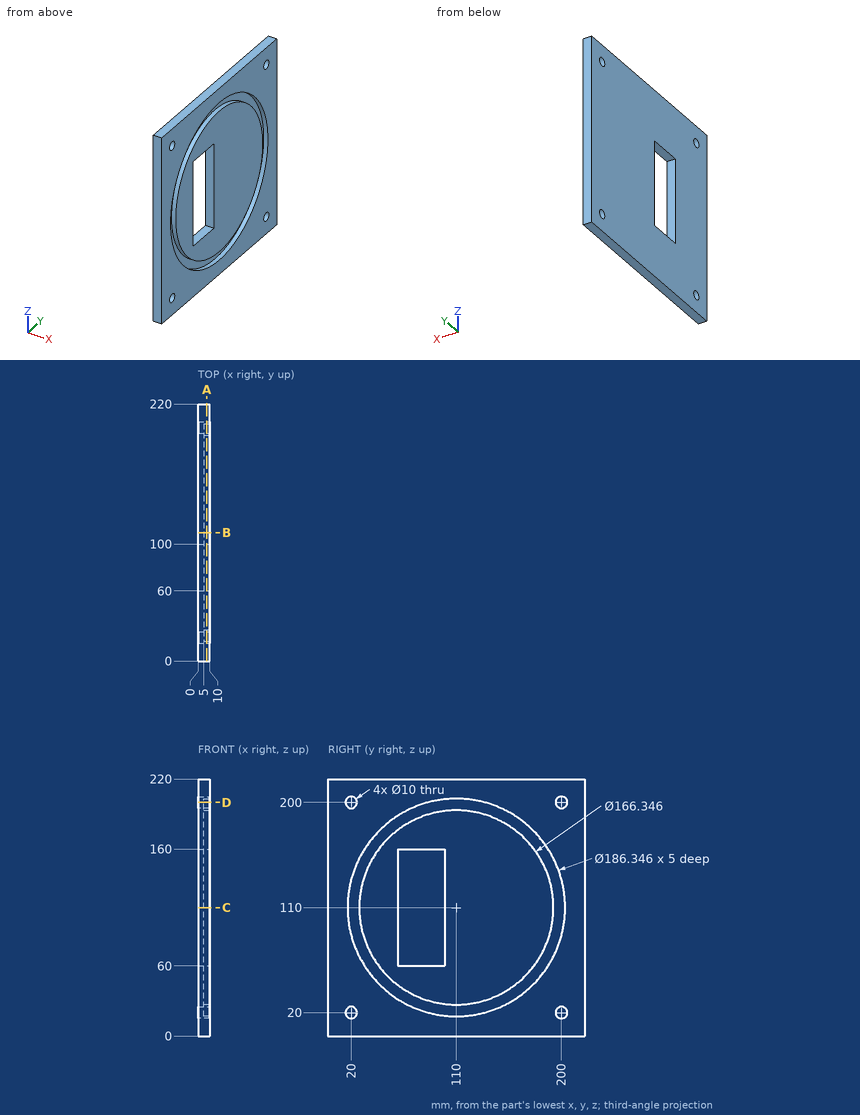
Input: dimensioned drawing with shaded views. Units: mm. Origin: part minimum x, y, z. Coordinates: 2 decimals unless noted, no trailing zeros. Order: outer loops, then holes, each group sorted by start corner. A loop starts at its lowest first (then second) coordinate and runs counter-clockwise, first axis right, second up.
1. Cut plane A-A, the plane x = 7.5. Return loops of the section in (y, z), plus the area to 3 significant figures.
Checked values:
outline: (0, 0) - (220, 0) - (220, 220) - (0, 220) - close; circle Ø166.35 at (110, 110); hole circle Ø10 at (20, 20); hole circle Ø10 at (20, 200); hole circle Ø186.35 at (110, 110); hole (60, 60) - (100, 60) - (100, 160) - (60, 160) - close; hole circle Ø10 at (200, 20); hole circle Ø10 at (200, 200)
area: 38,500 mm2
2. Cut plane C-C, the plane z = 110. Return loops of the section in (x, y), plus the area to 3 significant figures.
Checked values:
outline: (0, 0) - (10, 0) - (10, 16.83) - (5, 16.83) - (5, 26.83) - (10, 26.83) - (10, 60) - (0, 60) - close; (0, 100) - (10, 100) - (10, 193.17) - (5, 193.17) - (5, 203.17) - (10, 203.17) - (10, 220) - (0, 220) - close
area: 1,700 mm2
3. Cut plane D-D, the plane z = 200. Return loops of the section in (x, y), plus the area to 3 significant figures.
Checked values:
outline: (0, 0) - (10, 0) - (10, 15) - (0, 15) - close; (0, 25) - (10, 25) - (10, 85.89) - (5, 85.89) - (5, 134.11) - (10, 134.11) - (10, 195) - (0, 195) - close; (0, 205) - (10, 205) - (10, 220) - (0, 220) - close
area: 1,760 mm2
4. Cut plane B-B, the plane y = 110. Return loops of the section in (x, z), plus the area to 3 significant figures.
Checked values:
outline: (0, 0) - (10, 0) - (10, 16.83) - (5, 16.83) - (5, 26.83) - (10, 26.83) - (10, 193.17) - (5, 193.17) - (5, 203.17) - (10, 203.17) - (10, 220) - (0, 220) - close
area: 2,100 mm2
5. Ray query, line 1 along Y through (x, z) = (6.45, 110); line 2 along Z through (x, y) = (9.75, 112); line 3 along Y through (x, z) = (3.75, 144). Return the intervals inside material, ascending.
Checked values:
line 1: y = 0 to 16.83, 26.83 to 60, 100 to 193.17, 203.17 to 220
line 2: z = 0 to 16.85, 26.85 to 193.15, 203.15 to 220
line 3: y = 0 to 60, 100 to 220
